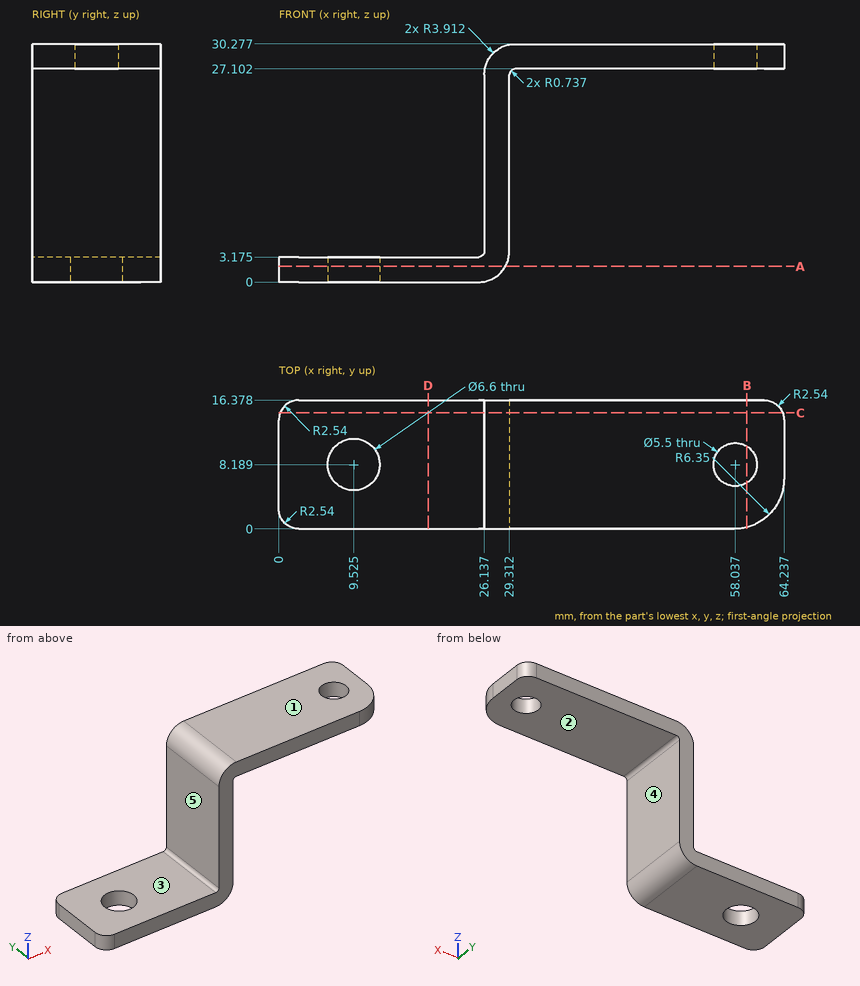
Job drawing, mm, ordinate dimensions from the low corner. One solid piece. A direction names the side the tool comes from. Give positions to 0.01 mm unless a question says otherwise; leave off trailing zeros. Write each loop counter-clockwise with the first axis right and the second up, starting at its lowest first coordinate (ties: lowest second). Pieces come first, ordered by that corner, then holes. Notation, with made-up numbers: (72, -31.75) -> (117, -31.75) arc R18 ccw to (117, -25.75) -> close; hole circle Ø10 at (49.25, 1). An arc over 180 degrees is marked (long way). Return JSON: item names as keys, results as strings.
Item 1: Drop flat-ended pins along their axis: pin 1 (5.5 mm diameter, centred on x = 9.525, y = 8.189, fed in from -Z); pin 2 (3 mm diameter, centred on x = 16.5, y = 2.5, fed in from +Z) (3 decimals); pin 3 (5 mm diameter, centred on y = 7.5, z = 10.5, fed in from +X). Give the stop position or say it passes through.
Answer below:
{"pin 1": "passes through", "pin 2": "stops at z = 3.175", "pin 3": "stops at x = 29.31"}
Item 2: Band-saw the part on B-B (x = 59.5). List the corners of the cut face in (y, z).
Answer below:
{"outline": "(0.21, 27.1) -> (5.86, 27.1) -> (5.86, 30.28) -> (0.21, 30.28) -> close; (10.52, 27.1) -> (16.38, 27.1) -> (16.38, 30.28) -> (10.52, 30.28) -> close"}
Item 3: Two-plate mould, pull along X, no slides. Class the marked faces 3, 4 and 5: +X half, -X half, draft (parallel to the pull), parting line (faces both ways), or undercut.
Answer below:
{"face 3": "draft", "face 4": "+X half", "face 5": "-X half"}
Item 4: Tool access for the marked faces 1 and 2: list every direction of +Z, -Z, +X, -X, +Y, -Y with a clear straight run to the whole face (end or side of a thin tool).
Answer below:
{"face 1": "+Z, +X, -X, +Y, -Y", "face 2": "-Z, +X, +Y, -Y"}
Item 5: Band-saw the part on C-C (y = 14.75). List the corners of the cut face in (x, z) (1 decimal).
Answer below:
{"outline": "(0.2, 0) -> (25.4, 0) arc R3.9 ccw to (29.3, 3.9) -> (29.3, 26.4) arc R0.7 cw to (30, 27.1) -> (64.1, 27.1) -> (64.1, 30.3) -> (30, 30.3) arc R3.9 ccw to (26.1, 26.4) -> (26.1, 3.9) arc R0.7 cw to (25.4, 3.2) -> (0.2, 3.2) -> close"}
Item 6: Drill centre lines: probe 1 along X at (y, z) = (7.25, 25.5); probe 2 along Z at (x, y) = (48.5, 12.25); probe 3 along Z at (x, y) = (7, 0.75) (1 decimal). Where is each one in solid material? Low to high.
Answer below:
{"probe 1": "x = 26.14 to 29.31", "probe 2": "z = 27.1 to 30.28", "probe 3": "z = 0 to 3.2"}
Item 7: Band-saw the part on D-D (x = 19). List the corners of the cut face in (y, z) (1 decimal).
Answer below:
{"outline": "(0, 0) -> (16.4, 0) -> (16.4, 3.2) -> (0, 3.2) -> close"}
Item 8: Band-saw the part on A-A (z = 2). List the corners of the cut face in (x, y) (1 decimal).
Answer below:
{"outline": "(0, 2.5) arc R2.5 ccw to (2.5, 0) -> (28.8, 0) -> (28.8, 16.4) -> (2.5, 16.4) arc R2.5 ccw to (0, 13.8) -> close; hole circle Ø6.6 at (9.5, 8.2)"}
